Input: part model. Units: mm. Frame: model coordinates. A direction names the side the tool comes from. Round coordinates to 2 decimals unless told otherwise and drop trailing zeros. Write each loop counter-clockwise with the first axis right and the second up, starting at its lowest first coordinate (ties: lowest second). Pieces come first, ordered by that corner, then holes. Notation, with made-up numbers: (84, -32.75) -> (93, -32.75) arc R23 ccw to (93, -11.75) -> close; hole circle Ø6 at (15.25, 72). An arc over 180 degrees is marked (long way). Write item = value, one per line. Start each with the question number.
```python
from build123d import *

# Parameters (mm, degrees)
SKETCH6_R                          = 15
BOSS_EXTRUDE3_DEPTH                = 12
CUT_EXTRUDE3_START                 = -2
SKETCH8_R                          = 11
CUT_EXTRUDE3_DEPTH                 = 8
F_6_0_6_DIAMETER_HOLE3_D           = 6
F_6_0_6_DIAMETER_HOLE3_ON_FACE_2_D = 6
F_6_0_6_DIAMETER_HOLE3_ON_FACE_3_D = 6


with BuildPart() as part:
    # Sketch6 → Boss-Extrude3 (new body)
    with BuildSketch(Plane(origin=(0, 0, 0), x_dir=(1, 0, 0), z_dir=(0, 1, 0))):
        Circle(SKETCH6_R)
    extrude(amount=BOSS_EXTRUDE3_DEPTH)

    # Sketch8 → Cut-Extrude3 (cut)
    with BuildSketch(Plane(origin=(0, 12, 0), x_dir=(1, 0, 0), z_dir=(0, 1, 0)).offset(CUT_EXTRUDE3_START)):
        Circle(SKETCH8_R)
    extrude(amount=-CUT_EXTRUDE3_DEPTH, mode=Mode.SUBTRACT)

    # Ø6.0 (6) Diameter Hole3 (through all)
    with Locations(Plane(origin=(13.257400922, 5.554097503, 7.017216029), x_dir=(-0.467814402, 0, 0.883826728), z_dir=(0.883826728, 0, 0.467814402))):
        with Locations((1e-09, 0)):
            Hole(F_6_0_6_DIAMETER_HOLE3_D / 2)

    # Ø6.0 (6) Diameter Hole3 on face 2 (through all)
    with Locations(Plane(origin=(13.269259555, 5.5012221, -6.994765961), x_dir=(0.466318067, 0, 0.884617127), z_dir=(0.884617127, 0, -0.466318067))):
        with Locations((0, 0)):
            Hole(F_6_0_6_DIAMETER_HOLE3_ON_FACE_2_D / 2)

    # Ø6.0 (6) Diameter Hole3 on face 3 (through all)
    with Locations(Plane(origin=(-4.253214755, 5.395471292, -14.384372223), x_dir=(-0.958958041, 0, 0.283548012), z_dir=(-0.283548012, 0, -0.958958041))):
        with Locations((0, 0)):
            Hole(F_6_0_6_DIAMETER_HOLE3_ON_FACE_3_D / 2)


solid = part.part
```
1. Line query: line 1 along Z through (x, y) = (0, 4.5); line 2 along Y through (x, z) = (0, 10). Output: solid intervals per line, ascending.
2. Section A-A (z = 0). Output: boundary loops of the cut face in (x, y), then the cut area to 3 significant figures.
3. Mould query, pull axis Z, two halves, no side actions, for faces 3 (the flat face through (0, 0, 0)), 4 (the cylindrical face through (-14.985, 5.916, -0.66)), 5 (the cylindrical face through (-12.738, 5.422, -3.351)). Classes: pulls with the +Z half, pulls with the -Z half, needs draft (parallel to the pull), parting line crosses it, or undercut.
4. Section B-B (y = 4.5). Output: boundary loops of the cut face in (x, z).
5. Reachability of faces 1 (the flat face through (0, 10, 0)), 2 (the flat face through (0, 12, 0)) from +Z, -Z, +X, -X, +Y, -Y: full face, straight path, thin tool, end or side. Return the list, or none.
6. Pin query (flat end, axial travel): P1, Ø6, axis at y = 5.5, z = 12, coming from the +X side; P2, Ø5, axis at x = -11.5, y = 6, coming from the -Z side; P3, Ø5, axis at x = -5.5, y = 6.5, coming from the +Z side. Return the tip coordinate at first contact, or that it passes through.
Check sheet entries:
q1.line_1 = -15 to -11, 11 to 15
q1.line_2 = 0 to 2, 10 to 12
q2.outline = (-15, 0) -> (15, 0) -> (15, 12) -> (-15, 12) -> close; hole (-11, 2) -> (11, 2) -> (11, 10) -> (-11, 10) -> close
q2.area = 184 mm2
q3.face_3 = needs draft
q3.face_4 = parting line crosses it
q3.face_5 = undercut
q4.outline = (-14.35, 4.37) arc R15 ccw to (-14.34, -4.41) -> (-10.71, -2.49) arc R11 cw to (-10.72, 2.46) -> close; (-11.71, -9.38) arc R15 ccw to (-6.92, -13.31) -> (-5.76, -9.37) arc R11 cw to (-8.09, -7.46) -> close; (-11.71, 9.37) -> (-8.08, 7.46) arc R11 cw to (0.27, 11) -> (1.43, 14.93) arc R15 ccw to start; (-1.43, -14.93) arc R15 ccw to (11.71, -9.37) -> (8.08, -7.46) arc R11 cw to (-0.27, -11) -> close; (5.76, 9.37) arc R11 cw to (8.09, 7.46) -> (11.71, 9.38) arc R15 ccw to (6.92, 13.31) -> close; (10.71, 2.49) arc R11 cw to (10.72, -2.46) -> (14.35, -4.37) arc R15 ccw to (14.34, 4.41) -> close
q5.face_1 = none
q5.face_2 = +Z, -Z, +X, -X, +Y
q6.P1 = 11.78
q6.P2 = -12
q6.P3 = 14.7
